Autodesk Inventor part; units mm, degrees
ref_plane "YZ Plane" through (0, 0, 0) normal (1, 0, 0) x (0, 1, 0)
ref_plane "XZ Plane" through (0, 0, 0) normal (0, 1, 0) x (-1, 0, 0)
ref_plane "XY Plane" through (0, 0, 0) normal (0, 0, 1) x (1, 0, 0)
sketch "Skizze1" plane through (0, 0, 0) normal (0, 1, 0) x (-1, 0, 0)
  line L0 (-6, 0) -> (6, 0)
  arc A0 (-4.5, 1.5) -> (-6, 0) centre (-4.5, 0) ccw
  line L1 (4.5, 1.5) -> (-4.5, 1.5)
  arc A1 (6, 0) -> (4.5, 1.5) centre (4.5, 0) ccw
  line L2 (3.0007, -2.9) -> (3.0007, 0)
  line L3 (2.0007, 0) -> (2.0007, -2.9)
  line L4 (2.0007, -2.9) -> (3.0007, -2.9)
  line L5 (3.0007, -2.9) -> (3.5007, -1.8564)
  line L6 (3.5007, -1.8564) -> (3.0007, -1.8564)
  line L7 (-1.7993, -2.9) -> (-1.7993, 0)
  line L8 (-2.7993, 0) -> (-2.7993, -2.9)
  line L9 (-2.7993, -2.9) -> (-1.7993, -2.9)
  line L10 (-3.2993, -1.8564) -> (-2.7993, -2.9)
  line L11 (-2.7993, -1.8564) -> (-3.2993, -1.8564)
  point P0 (0, 0)
  point P1 (0, 0)
  dimension "d0" = 3
  dimension "d1" = 3
  dimension "d2" = 1
  dimension "d3" = 1
  dimension "d4" = 154.4
  dimension "d5" = 154.4
  dimension "d7" = 0.5
  dimension "d8" = 3.8
  dimension "d9" = 2.9
  dimension "d10" = 9
  dimension "d12" = 5.8
  dimension "d13" = 0.5
  dimension "d14" = 2.9
  dimension "d15" = 4.5
  dimension "d16" = 0
extrude "Extrusion1" add sketch "Skizze1" along normal blind 8
equation "\"d1\" = d0"
equation "\"d3\" = d2"
equation "\"d5\" = d4"
equation "\"d13\" = d7"
properties part number "Misumi_Cable_Clip"
CAD build for the part. Positions are in the model's coordinates, mm. A direction names the side the tool comes from. Give positions to 0.01 mm unless a question says otherwise; leave off trailing zeros. Loops run counter-clockwise (first coordinate to the right, second up) from the corner with the lowest first, then second, coordinate; pieces in that order, holes last. Notation, with made-up numbers: M 61.5,4 L 94.5,4 A15 ccw 94.5,23 Z; hole C 34,30.5 d3. An arc over 180 degrees is marked long. Answer in a Markdown table with one row per item. Add a question column.
Item 1: Drop flat-ended pins along their axis: P1, Ø1, axis at y = 4, z = -2, coming from the +X side; P2, Ø1.9, axis at x = -1, y = 4, coming from the -Z side; P3, Ø1.4, axis at y = 4, z = -1, coming from the +X side. Give the stop position or say it passes through.
Item 2: Band-saw the part on B-B on y = 2. Give the cut face in (x, z), then the cut area to 3 significant figures.
Item 3: Probe probe 1 along X at (y, z) = (1.5, -0.45); probe 2 along Z at (x, y) = (0.25, 6); probe 3 along X at (y, z) = (2.5, -2.65). List the from-to ranges inside material, lowest first.
Item 4: Band-saw the part on C-C on x = 4.25. Give the cut face in (y, z), then the cut area to 3 significant figures.
Item 5: Band-saw the part on A-A on z = -1.45. Give the cut face in (x, y).
Item 6: Tool access for faces 4 (the face through (-4, 4, 0)), 5 (the face through (2.799, 4, -1)), 6 (the face through (1.799, 4, -1)): list every direction of +Z, -Z, +X, -X, +Y, -Y with a clear straight run to the whole face (end or side of a thin tool).
Item 7: Mould opens along Z. For faces 1 (the face through (-3.247, 3.944, -2.386)), 2 (the face through (0.1, 0, 0.3)), 3 (the face through (-3.001, 4, -1)) say: +Z half, -Z half, draft (parallel to the pull), parting line (faces both ways), or undercut.
Item 8: Band-saw the part on D-D on z = -2.3. Give the cut face in (x, y), then the cut area to 3 significant figures.
Reply:
| question | item | result |
|---|---|---|
| 1 | P1 | stops at x = 3.3 |
| 1 | P2 | stops at z = 0 |
| 1 | P3 | stops at x = 2.8 |
| 2 | outline | M -6,0 L -3,0 L -3,-1.86 L -3.5,-1.86 L -3,-2.9 L -2,-2.9 L -2,0 L 1.8,0 L 1.8,-2.9 L 2.8,-2.9 L 3.3,-1.86 L 2.8,-1.86 L 2.8,0 L 6,0 A1.5 ccw 4.5,1.5 L -4.5,1.5 A1.5 ccw Z |
| 2 | area | 23.4 mm^2 |
| 3 | probe 1 | x = -3 to -2, 1.8 to 2.8 |
| 3 | probe 2 | z = 0 to 1.5 |
| 3 | probe 3 | x = -3.12 to -2, 1.8 to 2.92 |
| 4 | outline | M 0,0 L 8,0 L 8,1.5 L 0,1.5 Z |
| 4 | area | 12.0 mm^2 |
| 5 | outline | M -3,0 L -2,0 L -2,8 L -3,8 Z; M 1.8,0 L 2.8,0 L 2.8,8 L 1.8,8 Z |
| 6 | face 4 | -X, +Y, -Y |
| 6 | face 5 | +X, +Y, -Y |
| 6 | face 6 | -Z, +Y, -Y |
| 7 | face 1 | -Z half |
| 7 | face 2 | draft |
| 7 | face 3 | undercut |
| 8 | outline | M -3.29,0 L -2,0 L -2,8 L -3.29,8 Z; M 1.8,0 L 3.09,0 L 3.09,8 L 1.8,8 Z |
| 8 | area | 20.6 mm^2 |
